Geometry check sheet. Reference: the model listing, model coordinates, mm. Give positions to 0.01 mm unless a question says otherwise; leave off trailing zeros. Order: outer loops, then holes, each group sorted by start corner. A loop starts at its lowest first (then second) coordinate and runs counter-clockwise, first axis right, second up. Notation, with made-up numbers: M 32,73.5 L 48,73.5 A35 ccw 48,110.5 Z; hole C 4,11.5 d9. An arc over 180 degrees is marked long. Answer as a JSON object with one key per item and string values. Group by question number.
Autodesk Inventor part; units mm, degrees
ref_plane "YZ Plane" through (0, 0, 0) normal (1, 0, 0) x (0, 1, 0)
ref_plane "XZ Plane" through (0, 0, 0) normal (0, 1, 0) x (-1, 0, 0)
ref_plane "XY Plane" through (0, 0, 0) normal (0, 0, 1) x (1, 0, 0)
sketch "Sketch1" plane through (0, 0, 0) normal (0, 0, 1) x (1, 0, 0)
  circle A0 centre (0, 0) radius 4.25
  dimension "d0" = 8.5
extrude "Extrusion1" add sketch "Sketch1" along normal mid plane 100
sketch "Sketch2" plane through (0, 0, 50) normal (0, 0, 1) x (1, 0, 0)
  circle A0 centre (0, 0) radius 6
  dimension "d3" = 12
extrude "Extrusion2" add sketch "Sketch2" along normal blind 5
mirror "Mirror1" about plane through (0, 0, 0) normal (0, 0, 1) of "Extrusion2"
fillet "Fillet1" radius 0.5 4 edges at (-6, 0, -55) (-6, 0, -50) (-6, 0, 55) (-6, 0, 50)
properties part number "Connecting rod hinge" material "Stainless Steel"
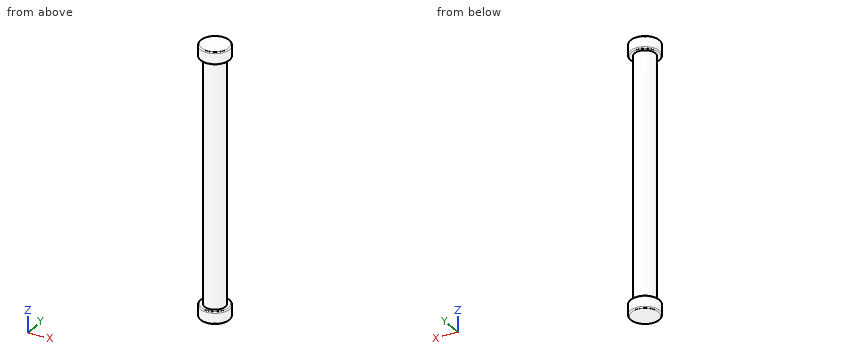
1. Cross-section at A-A (x = 0). Record the cut outline in (y, z).
2. Cross-section at C-C (z = -16). Record the cut outline in (x, y), and give its area (3 significant figures).
3. Depth check by flat-ended pin: pin 1 (1.5 mm diameter, centred on y = 2.5, z = 29.5, fed in from +X); pin 2 (6 mm diameter, centred on y = 2.5, z = -9, fed in from +X); pin 3 (6 mm diameter, centred on x = 3.5, z = -12, fed in from +Y); pin 4 (2 mm diameter, centred on x = 5, y = 4, fed in from -Z). Enter the tip coordinate at first touch or a pass-through.
4. Thickness scan on line 1 along Z through (x, y) = (-5.5, -1); line 2 along X through (y, z) = (2.25, -42); line 3 along Y through (x, z) = (-1.25, -2.5). Record the ranges inside material, lowest first. Write a range as [from, to].
Report:
{
 "1": {"outline": "M -6,-54.5 A0.5 ccw -5.5,-55 L 5.5,-55 A0.5 ccw 6,-54.5 L 6,-50.5 A0.5 ccw 5.5,-50 L 4.25,-50 L 4.25,50 L 5.5,50 A0.5 ccw 6,50.5 L 6,54.5 A0.5 ccw 5.5,55 L -5.5,55 A0.5 ccw -6,54.5 L -6,50.5 A0.5 ccw -5.5,50 L -4.25,50 L -4.25,-50 L -5.5,-50 A0.5 ccw -6,-50.5 Z"},
 "2": {"outline": "C 0,0 d8.5", "area": "56.7 mm2"},
 "3": {"pin 1": "stops at x = 3.87", "pin 2": "stops at x = 4.25", "pin 3": "stops at y = 4.22", "pin 4": "stops at z = -55"},
 "4": {"line 1": "z = [-54.99, -50.01], [50.01, 54.99]", "line 2": "x = [-3.61, 3.61]", "line 3": "y = [-4.06, 4.06]"}
}
